from build123d import *

# Parameters (mm, degrees)
SKETCH_1_W          = 18
SKETCH_1_H          = 12.5
EXTRUDE_1_DEPTH     = 8
SKETCH_2_R          = 1.625
CUT_EXTRUDE_1_DEPTH = 2.5
EXTRUDE_START       = 1
SKETCH_3_R          = 2.5
SKETCH_3_R_2        = 1.625
EXTRUDE_2_DEPTH     = 1
SKETCH_4_R          = 1.25
CUT_EXTRUDE_2_DEPTH = 25
FILLET_1_R          = 4
FILLET_2_R          = 2
CUT_EXTRUDE_3_DEPTH = 2
SKETCH_6_R          = 1.65
SKETCH_6_R_2        = 1.7
CUT_EXTRUDE_4_DEPTH = 8


with BuildPart() as part:
    # 草图1 → 凸台-拉伸1 (new body)
    with BuildSketch(Plane.XY):
        Rectangle(SKETCH_1_W, SKETCH_1_H)
    extrude(amount=EXTRUDE_1_DEPTH)

    # 草图2 → 切除-拉伸1 (cut, symmetric)
    with BuildSketch(Plane(origin=(0, 0, 0), x_dir=(-1, 0, 0), z_dir=(0, 0, -1))):
        with Locations((0, 1.45)):
            Circle(SKETCH_2_R)
    extrude(amount=CUT_EXTRUDE_1_DEPTH, both=True, mode=Mode.SUBTRACT)

    # 草图3 → 凸台-拉伸2 (add)
    with BuildSketch(Plane(origin=(0, 0, 0), x_dir=(-1, 0, 0), z_dir=(0, 0, -1)).offset(EXTRUDE_START)):
        with Locations(Location((0, 1.45, 0), (0, 0, 180))):
            Circle(SKETCH_3_R)
        with Locations((0, 1.45)):
            Circle(SKETCH_3_R_2, mode=Mode.SUBTRACT)
    extrude(amount=-EXTRUDE_2_DEPTH)

    # 草图4 → 切除-拉伸2 (cut)
    with BuildSketch(Plane(origin=(0, 6.25, 0), x_dir=(1, 0, 0), z_dir=(0, 1, 0))):
        with Locations(Location((-5.5, -4, 0), (0, 0, 270))):
            Circle(SKETCH_4_R)
    cut_extrude_2 = extrude(amount=-CUT_EXTRUDE_2_DEPTH, mode=Mode.SUBTRACT)

    # 镜向1: 切除-拉伸2 across plane
    add(cut_extrude_2.mirror(Plane(origin=(0, 0, 0), x_dir=(0, 0, 1), z_dir=(1, 0, 0))), mode=Mode.SUBTRACT)

    # 圆角1
    fillet_1_edges = [part.edges().sort_by_distance(p)[0] for p in [
        (-9, 0, 8),
        (9, 0, 8),
    ]]
    fillet(fillet_1_edges, radius=FILLET_1_R)

    # 圆角2
    fillet_2_edges = [part.edges().sort_by_distance(p)[0] for p in [
        (-9, 0, 0),
        (9, 0, 0),
    ]]
    fillet(fillet_2_edges, radius=FILLET_2_R)

    # 草图5 → 切除-拉伸3 (cut)
    with BuildSketch(Plane(origin=(0, 6.25, 0), x_dir=(1, 0, 0), z_dir=(0, 1, 0))):
        with BuildLine():
            Line((7, 0), (-7, 0))
            ThreePointArc((-7, 0), (-8.414213562, -0.585786438), (-9, -2))
            Line((-9, -2), (-9, -4))
            ThreePointArc((-9, -4), (-7.828427125, -6.828427125), (-5, -8))
            Line((-5, -8), (5, -8))
            ThreePointArc((5, -8), (7.828427125, -6.828427125), (9, -4))
            Line((9, -4), (9, -2))
            ThreePointArc((9, -2), (8.414213562, -0.585786438), (7, 0))
        make_face()
    extrude(amount=-CUT_EXTRUDE_3_DEPTH, mode=Mode.SUBTRACT)

    # 草图6 → 切除-拉伸4 (cut)
    with BuildSketch(Plane(origin=(0, 4.25, 0), x_dir=(1, 0, 0), z_dir=(0, 1, 0))):
        with Locations(Location((5.5, -4, 0), (0, 0, 270))):
            Circle(SKETCH_6_R)
        with Locations(Location((-5.5, -4, 0), (0, 0, 270))):
            Circle(SKETCH_6_R_2)
    extrude(amount=-CUT_EXTRUDE_4_DEPTH, mode=Mode.SUBTRACT)


solid = part.part
Source: CAD feature listing. Evaluate the final solid. Frame: model axes, mm. A direction names the side the tool comes from. Give positions to 0.01 mm unless a question says otherwise; leave off trailing zeros. Loops run counter-clockwise (first coordinate to the right, second up) from the corner with the lowest first, then second, coordinate; pieces in that order, holes last. Notation, with made-up numbers: (-39, 78.25) -> (-9, 78.25) arc R25 ccw to (-9, 92.25) -> close; hole circle Ø4 at (-29, 13.5). An arc over 180 degrees is marked (long way). Use a Markdown table: item, result. Add a question column.
1) Section query D-D, the plane z = 1. Return the cut outline in (x, y) (3 decimals).
2) Section query B-B, the plane x = -5.5. Return the cut outline in (y, z).
3) Line query: line 1 along X through (y, z) = (2.5, 4); line 2 along X through (y, z) = (-4.5, 4); line 3 along Z through (x, y) = (-3, 1.5). Output: solid intervals per line, ascending. Write a range as [from, to].
4) First-contact query: pin 1 (1.5 mm diameter, centred on y = 1, z = 5.5, fed in from -X); pin 2 (5 mm diameter, centred on y = -4.5, z = 7, fed in from -X); pin 3 (3 mm diameter, centred on x = -5.5, z = 4, fed in from +Y). Flat tips, straight axial feed; report the tip coordinate or a pass-through.
5) Pull-direction query (Y, two-part tool) for faces 4 (the face through (6.609, -4.982, 4.577)), 5 (the face through (1.29, 0.46, 0.73)), 6 (the face through (0, 4.25, 4)); classes: +Y half, -Y half, draft (parallel to the pull), parting line (faces both ways), or undercut.
6) Section query A-A, the plane y = -5.5. Return the cut outline in (x, z).
7) Section query C-C, the plane z = 5. Return the cut outline in (x, y), then the cut area to 3 significant figures.
8) Reachability of faces 1 (the face through (-0.33, -1.03, -0.51)), 2 (the face through (-7.859, -0.926, 6.797)), 3 (the face through (3.9, 0.3, 3.6)) from +Z, -Z, +X, -X, +Y, -Y: full face, straight path, thin tool, end or side. Return the list, or none.
Numbers:
| question | item | result |
|---|---|---|
| 1 | outline | (-8.732, -6.25) -> (8.732, -6.25) -> (8.732, 4.25) -> (-8.732, 4.25) -> close; hole circle Ø3.25 at (0, 1.45) |
| 2 | outline | (-6.25, 0) -> (4.25, 0) -> (4.25, 2.3) -> (-3.75, 2.3) -> (-3.75, 2.75) -> (-6.25, 2.75) -> close; (-6.25, 5.25) -> (-3.75, 5.25) -> (-3.75, 5.7) -> (4.25, 5.7) -> (4.25, 7.97) -> (-6.25, 7.97) -> close |
| 3 | line 1 | x = [-9, -7.2], [-3.8, 3.85], [7.15, 9] |
| 3 | line 2 | x = [-9, -6.75], [-4.25, 4.25], [6.75, 9] |
| 3 | line 3 | z = [0, 8] |
| 4 | pin 1 | stops at x = -8.93 |
| 4 | pin 2 | stops at x = -8.97 |
| 4 | pin 3 | stops at y = -3.75 |
| 5 | face 4 | draft |
| 5 | face 5 | undercut |
| 5 | face 6 | +Y half |
| 6 | outline | (-9, 2) arc R2 ccw to (-7, 0) -> (7, 0) arc R2 ccw to (9, 2) -> (9, 4) arc R4 ccw to (5, 8) -> (-5, 8) arc R4 ccw to (-9, 4) -> close; hole circle Ø2.5 at (-5.5, 4); hole circle Ø2.5 at (5.5, 4) |
| 7 | outline | (-8.87, -6.25) -> (-6.25, -6.25) -> (-6.25, -3.75) -> (-6.87, -3.75) -> (-6.87, 4.25) -> (-8.87, 4.25) -> close; (-4.75, -6.25) -> (4.75, -6.25) -> (4.75, -3.75) -> (4.19, -3.75) -> (4.19, 4.25) -> (-4.13, 4.25) -> (-4.13, -3.75) -> (-4.75, -3.75) -> close; (6.25, -6.25) -> (8.87, -6.25) -> (8.87, 4.25) -> (6.81, 4.25) -> (6.81, -3.75) -> (6.25, -3.75) -> close |
| 7 | area | 136 mm2 |
| 8 | face 1 | -Z |
| 8 | face 2 | +Z, -X, +Y, -Y |
| 8 | face 3 | +Y |
